Autodesk Inventor part; units mm, degrees
ref_plane "Płaszczyzna konstrukcyjna2" through (-6, 5, 0) normal (0, 0, 1) x (1, 0, 0)
ref_plane "YZ Plane" through (0, 0, 0) normal (1, 0, 0) x (0, 1, 0)
ref_plane "XZ Plane" through (0, 0, 0) normal (0, 1, 0) x (-1, 0, 0)
sketch "Szkic3" plane through (0, 0, 0) normal (0, 1, 0) x (-1, 0, 0)
  circle A0 centre (0, 0) radius 5
  line L0 (-6, -6) -> (6, -6)
  line L1 (6, -6) -> (6, 6)
  line L2 (6, 6) -> (-6, 6)
  line L3 (-6, 6) -> (-6, -6)
  line L4 (-6, -6) -> (6, 6) construction
  line L5 (6, -6) -> (-6, 6) construction
  dimension "d12" = 10
  dimension "d15" = 12
  dimension "d16" = 12
extrude "Wyciągnięcie proste3" add sketch "Szkic3" along normal mid plane 10
extrude "Wyciągnięcie proste4" add sketch "Szkic3" along normal blind 5 contours A0
ref_plane "Płaszczyzna konstrukcyjna2" through (-6, 5, 0) normal (0, 0, 1) x (1, 0, 0)
sketch "Szkic7" plane through (-6, 5, 0) normal (0, 0, 1) x (1, 0, 0)
  line L0 (0, 0) -> (12, 0)
  line L1 (0, 0) -> (12, 0)
  line L2 (6, 0) -> (6, 6)
  line L3 (6, 0) -> (12, 0) construction
  circle A0 centre (6, 6) radius 2
  line L4 (4.2679, 5) -> (3.2679, 5)
  line L5 (6, 8) -> (6, 9)
  line L6 (7.7321, 5) -> (8.7321, 5)
  arc A1 (0, 0) -> (3.2679, 5) centre (-8.0948, 8.8586) ccw
  arc A2 (6, 9) -> (3.2679, 5) centre (6.0958, 6.0015) ccw
  arc A3 (8.7321, 5) -> (6, 9) centre (5.9042, 6.0015) ccw
  arc A4 (8.7321, 5) -> (12, 0) centre (20.0948, 8.8586) ccw
  point P0 (6, -5)
  dimension "d42" = 6
  dimension "d43" = 90
  dimension "d44" = 4
  dimension "d45" = 1
  dimension "d46" = 1
  dimension "d47" = 1
  dimension "d48" = 5
  dimension "d49" = 5
  dimension "d50" = 0
  dimension "d51" = 12
  dimension "d52" = 3
  dimension "d53" = 3
  dimension "d54" = 12
extrude "Wyciągnięcie proste7" add sketch "Szkic7" along normal mid plane 4 contours A1 L4 A0 L2 L0 | L2 A0 L6 A4 L0 | A2 L5 A0 L4 | A3 L6 A0 L5
fillet "Zaokrąglenie5" radius 6 4 edges at (-6, 5, 4) (6, 5, 4) (6, 5, -4) (-6, 5, -4)
fillet "Zaokrąglenie6" radius 6 2 edges at (6, 5, 0) (-6, 5, 0)
properties part number "Connector_fill"
Build history of the part. All positions in model axes, mm. A direction names the side the tool comes from. Coordinates: 2 decimals unless noted, no trailing zeros. Order: outer loops, then holes, each group sorted by start corner. A loop starts at its lowest first (then second) coordinate and runs counter-clockwise, first axis right, second up. Notation, with made-up numbers: (-5.75, 47.25) - (1.25, 47.25) arc R11 ccw to (1.25, 59.25) - close; hole circle Ø7 at (71.5, -12). An arc over 180 degrees is marked (long way). Write item = value, one per line. Start each with the question number.
1) Saw through at C-C on x = -1. Write the cut outline in (y, z), then the cut area to 3 significant figures.
2) Two-plate mould, pull along Z, no slides. Class faces 1 (the face through (0, 0, 0)), 2 (the face through (0, 7, -2)), 3 (the face through (-2.404, 12.661, -0.028)): pulls with the +Z half, pulls with the -Z half, needs draft (parallel to the pull), parting line crosses it, or undercut.
3) 3-axis set-ups, long thin cutter, end or side, ignore diameter. For faces 4 (the face through (-4.196, 3.289, -3.972)), 5 (the face through (-4.196, 3.289, 4.028)), 6 (the face through (4.196, 3.289, 3.972)): which of +Z, -Z, +X, -X, +Y, -Y reach the whole face in a straight line?
4) Saw through at B-B on z = 0. Write the cut outline in (x, y), then the cut area to 3 significant figures.
5) Flat gauge pins, fed straight in: pin 1 Ø3 at (x, z) = (-4, -1) entering from -Y; pin 2 Ø1.5 at (x, z) = (-2.5, 2.5) entering from -Y; pin 3 Ø1 at (x, y) = (-1, 9) entering from -Z; pin 4 Ø5 at (y, z) = (10, -0.5) entering from -X. Where does each tip first touch, or does it go through?
6) Wall check: line 1 along Z through (x, y) = (0, -3); line 2 along X through (y, z) = (11, 1.1); line 3 along Y through (x, z) = (0, -0.7). Give the ranges that are in metal, low to high. Write a range as from..to.
7) Saw through at A-A on y = 11. Write the cut outline in (x, z), then the cut area to 3 significant figures.
From the geometry:
q1.outline = (-5, -6) - (4.92, -6) - (4.92, -2) - (9.27, -2) - (9.27, 2) - (4.92, 2) - (4.92, 6) - (-5, 6) - (-5, 4.9) - (0, 4.9) - (0, -4.9) - (-5, -4.9) - close; (12.73, -2) - (13.79, -2) - (13.79, 2) - (12.73, 2) - close
q1.area = 91.7 mm^2
q2.face_1 = undercut
q2.face_2 = pulls with the -Z half
q2.face_3 = needs draft
q3.face_4 = -Z, -X, +Y
q3.face_5 = +Z, -X, +Y
q3.face_6 = +Z, +X, +Y
q4.outline = (-6, -5) - (-5, -5) - (-5, 0) - (5, 0) - (5, -5) - (6, -5) - (6, 2.66) arc R6 ccw to (4.7, 6.39) arc R12 cw to (2.73, 10) arc R3 ccw to (0, 14) arc R3 ccw to (-2.73, 10) arc R12 cw to (-4.7, 6.39) arc R6 ccw to (-6, 2.66) - close; hole circle Ø4 at (0, 11)
q4.area = 116 mm^2
q5.pin_1 = -5
q5.pin_2 = 0
q5.pin_3 = -2
q5.pin_4 = -3.92
q6.line_1 = -6..-5, 5..6
q6.line_2 = -2.9..-2, 2..2.9
q6.line_3 = 0..9, 13..14
q7.outline = (-2.9, -2) - (-2, -2) - (-2, 2) - (-2.9, 2) - close; (2, -2) - (2.9, -2) - (2.9, 2) - (2, 2) - close
q7.area = 7.23 mm^2
